```python
from build123d import *

# Parameters (mm, degrees)
F0_W        = 41
F0_H        = 4
F1_DEPTH    = 6
F3_START    = -6.6
F2_R        = 3.4
F3_DEPTH    = 7.4
F4_T1_DEPTH = 37
F4_T3_DEPTH = 36.4948974279
F4_T5_DEPTH = 7.4
F4_T7_DEPTH = 7.4
F5_DEPTH    = 17
F6_R        = 10
F7_R        = 1.99999
F8_R        = 2
F2_R_2      = 1.75
F9_DEPTH    = 18.001


# Not quite as in the source:
# - a fillet or chamfer that OpenCascade refuses, or shapes differently, is made with other operations: its cross-section is extruded or revolved along the edge and cut away or added
# - a fillet or chamfer is up to 0.001 mm smaller than in the source, because OpenCascade refuses the exact size


with BuildPart() as f1:
    # F0 (on Top) → F1 (new body, symmetric)
    with BuildSketch(Plane.XY):
        Polygon((11, -4.5), (21, -4.5), (21, 9.5), (-30, 9.5), (-30, 5), (-21.4, 5), (-21.4, 0), (-30, 0), (-30, -4.5), align=None)
        with Locations((-9.5, -6.5)):
            Rectangle(F0_W, F0_H)
    extrude(amount=F1_DEPTH, both=True)

    # F2 (on face) → F3 (cut)
    with BuildSketch(Plane.XZ.offset(8.5).offset(F3_START)):
        with BuildLine():
            Line((11, -5.9371710435), (11, 5.9371710435))
            ThreePointArc((11, 5.9371710435), (10.9829729772, 5.9686099372), (10.9658560997, 6))
            Line((10.9658560997, 6), (-10.9658560997, 6))
            ThreePointArc((-10.9658560997, 6), (-12.5, 0), (-10.9658560997, -6))
            Line((-10.9658560997, -6), (10.9658560997, -6))
            ThreePointArc((10.9658560997, -6), (10.9829729772, -5.9686099372), (11, -5.9371710435))
        make_face()
        Circle(F2_R, mode=Mode.SUBTRACT)
        with BuildLine():
            ThreePointArc((11, -5.9371710435), (12.1191996435, -3.0618621785), (12.5, 0))
            ThreePointArc((12.5, 0), (12.1191996435, 3.0618621785), (11, 5.9371710435))
            Line((11, 5.9371710435), (11, -5.9371710435))
        make_face()
        Circle(F2_R)
    extrude(amount=-F3_DEPTH, mode=Mode.SUBTRACT)

    # F4: fillet of radius 5 on 4 edges, made by hand

    # F4_s2 → F4_t1 (cut)
    with BuildSketch(Plane.XY.offset(-18.5)):
        with BuildLine():
            ThreePointArc((-25, -8.5), (-28.5355339059, -7.0355339059), (-30, -3.5))
            Line((-30, -3.5), (-30, -8.5))
            Line((-30, -8.5), (-25, -8.5))
        make_face()
    extrude(amount=F4_T1_DEPTH, mode=Mode.SUBTRACT)

    # F4_s4 → F4_t3 (cut)
    with BuildSketch(Plane.XY.offset(-18.2474487139)):
        with BuildLine():
            ThreePointArc((11, -4.5), (9.2632981746, -7.3729833462), (6.1010205144, -8.5))
            Line((6.1010205144, -8.5), (11, -8.5))
            Line((11, -8.5), (11, -4.5))
        make_face()
    extrude(amount=F4_T3_DEPTH, mode=Mode.SUBTRACT)

    # F4_s6 → F4_t5 (cut)
    with BuildSketch(Plane.XZ.offset(-5.5)):
        with BuildLine():
            ThreePointArc((-17.4714052097, 6), (-13.8362593097, 4.4330328116), (-12.4795751498, 0.7142857143))
            ThreePointArc((-12.4795751498, 0.7142857143), (-12.0169361942, 3.4414015319), (-10.9658560997, 6))
            Line((-10.9658560997, 6), (-17.4714052097, 6))
        make_face()
    extrude(amount=F4_T5_DEPTH, mode=Mode.SUBTRACT)

    # F4_s8 → F4_t7 (cut)
    with BuildSketch(Plane.XZ.offset(-5.5)):
        with BuildLine():
            ThreePointArc((17.4714052097, 6), (13.8362593097, 4.4330328116), (12.4795751498, 0.7142857143))
            ThreePointArc((12.4795751498, 0.7142857143), (12.0169361943, 3.4414015319), (10.9658560997, 6))
            Line((10.9658560997, 6), (17.4714052097, 6))
        make_face()
    extrude(amount=F4_T7_DEPTH, mode=Mode.SUBTRACT)

    # F2 (on face) → F5 (cut, through all)
    with BuildSketch(Plane.XZ.offset(8.5)):
        Circle(F2_R)
    extrude(amount=-F5_DEPTH, mode=Mode.SUBTRACT)

    # F6
    f6_edges = [f1.edges().sort_by_distance(p)[0] for p in [
        (21, 2.5, -6),
    ]]
    fillet(f6_edges, radius=F6_R)

    # F7 (radius 2 in the source; OpenCascade refuses exactly that, so slightly less here)
    f7_edges = [f1.edges().sort_by_distance(p)[0] for p in [
        (21, 2.5, 6),
    ]]
    fillet(f7_edges, radius=F7_R)

    # F8
    f8_edges = [f1.edges().sort_by_distance(p)[0] for p in [
        (-30, 9.5, 0),
        (-21.4, 5, 0),
        (-21.4, 0, 0),
    ]]
    fillet(f8_edges, radius=F8_R)

    # F2 (on face) → F9 (cut, through all)
    with BuildSketch(Plane.XZ.offset(8.5)):
        with Locations((15.5, 0.25)):
            Circle(F2_R_2)
    extrude(amount=-F9_DEPTH, mode=Mode.SUBTRACT)


solid = f1.part
```
Can you work these out from the model? Positions are in its coordinate system, mm. A direction names the side the tool comes from. Coordinates: 2 decimals unless noted, no trailing zeros. Order: outer loops, then holes, each group sorted by start corner. A loop starts at its lowest first (then second) coordinate and runs counter-clockwise, first axis right, second up. Notation, with made-up numbers: (72.5, -19) - (87.5, -19) arc R22 ccw to (87.5, -4) - close; hole circle Ø3 at (21, 75.5). An arc over 180 degrees is marked (long way). Answer in a Markdown table with one row per item.
1. Suppose I cut it at C-C (x = 16). Please give me the cut outline in (y, z), and give its area (3 significant figures).
Reply:
| item | result |
|---|---|
| outline | (-4.5, -4.66) - (9.5, -4.66) - (9.5, -1.43) - (-4.5, -1.43) - close; (-4.5, 1.93) - (9.5, 1.93) - (9.5, 6) - (5.5, 6) - (5.5, 5.78) - (-1.9, 5.78) - (-1.9, 6) - (-4.5, 6) - close |
| area | 101 mm^2 |
2. If I drill on line 1 along Z through (x, y) = (0, 7.3); line 2 along Y through (x, z) = (-24.5, -5); line 3 along X through (y, z) = (-1, -1), over which ranges is the centre line in solid material (lowest first)?
Reply:
| item | result |
|---|---|
| line 1 | z = -6 to -3.4, 3.4 to 6 |
| line 2 | y = -8.5 to 0, 5 to 9.5 |
| line 3 | x = -30 to -12.46, 12.46 to 14.28, 16.72 to 19.66 |
3. For pin 1 (4 mm diameter, centred on y = 4.5, z = 0.5, fed in from -X); pin 2 (4 mm diameter, centred on x = 15.5, z = 0.25, fed in from -Y); pin 3 (0.5 mm diameter, centred on y = 2.5, z = -0.5, fed in from -X); pin 4 (4 mm diameter, centred on y = 1, z = 0, fed in from +X), each with a flat end and sliding along its axis, tell me the tip position at first contact or that it passes through.
Reply:
| item | result |
|---|---|
| pin 1 | stops at x = -30 |
| pin 2 | stops at y = -4.5 |
| pin 3 | stops at x = -21.4 |
| pin 4 | stops at x = 20.8 |
4. Suppose I cut it at A-A (x = 0). Please give me the cut outline in (y, z), and give its area (3 significant figures).
Reply:
| item | result |
|---|---|
| outline | (-8.5, -6) - (-1.9, -6) - (-1.9, -3.4) - (-8.5, -3.4) - close; (-8.5, 3.4) - (-1.9, 3.4) - (-1.9, 6) - (-8.5, 6) - close; (5.5, -6) - (9.5, -6) - (9.5, 6) - (5.5, 6) - (5.5, 3.4) - (8.5, 3.4) - (8.5, -3.4) - (5.5, -3.4) - close |
| area | 61.9 mm^2 |
5. Suppose I cut it at B-B (y = -1). Give the number of separate pieces and of enclosed holes in the cut face, and give its area (3 significant figures).
Reply:
| item | result |
|---|---|
| separate pieces | 2 |
| enclosed holes | 1 |
| area | 276 mm^2 |
6. If we mould it in two halves opening along X, with no side actions, what happens to faces 4 (the cylindrical face through (20.43, 2.6, 5.4)), 5 (the flat face through (-30, -2, 0)), 6 (the flat face through (-14, 1, -6)), 7 (the flat face through (0, 8.5, 0))? For each: pulls with the +X half, pulls with the -X half, needs draft (parallel to the pull), parting line crosses it, or undercut.
Reply:
| item | result |
|---|---|
| face 4 | pulls with the +X half |
| face 5 | pulls with the -X half |
| face 6 | needs draft |
| face 7 | undercut |
7. For faces 1 (the cylindrical face through (9.3, -7.342, -0.084)), 2 (the cylindrical face through (-21.97, 0.6, 0.08)), 3 (the flat face through (4, -1.9, 0)), which set-ups out of +Z, -Z, +X, -X, +Y, -Y let a thin tool reach every point of the face, with its end or its side?
Reply:
| item | result |
|---|---|
| face 1 | +Z, -Z, +X, -Y |
| face 2 | +Z, -Z, -X |
| face 3 | +Z |
